Autodesk Inventor part; units mm, degrees
ref_plane "YZ Plane" through (0, 0, 0) normal (1, 0, 0) x (0, 1, 0)
ref_plane "XZ Plane" through (0, 0, 0) normal (0, 1, 0) x (-1, 0, 0)
ref_plane "XY Plane" through (0, 0, 0) normal (0, 0, 1) x (1, 0, 0)
sketch "Sketch1" plane through (0, 0, 0) normal (0, 1, 0) x (-1, 0, 0)
  line L0 (0, 0) -> (-425, 0)
  line L1 (-425, 0) -> (-425, -355)
  line L2 (-425, -355) -> (0, -355)
  line L3 (0, -355) -> (0, 0)
  line L4 (-20, -15) -> (-405, -15)
  line L5 (-405, -15) -> (-405, -340)
  line L6 (-405, -340) -> (-20, -340)
  line L7 (-20, -340) -> (-20, -15)
  dimension "d0" = 425
  dimension "d1" = 355
  dimension "d2" = 385
  dimension "d3" = 325
extrude "Extrusion1" add sketch "Sketch1" along normal blind 247
sketch "Sketch2" plane through (0, 0, 0) normal (0, -1, 0) x (1, 0, 0)
  line L0 (0, -355) -> (0, 0)
  line L1 (425, 0) -> (425, -355)
  line L2 (0, 0) -> (425, 0)
  line L3 (425, 0) -> (425, -355)
  line L4 (425, -355) -> (0, -355)
  line L5 (0, -355) -> (0, 0)
extrude "Extrusion2" add sketch "Sketch2" against normal blind 7
sketch "Sketch3" plane through (20, 247, -15) normal (1, 0, 0) x (0, 0, -1)
  line L0 (0, -240) -> (325, -240)
  line L1 (0, -240) -> (162.5, -240)
  point P0 (-15, -247)
  dimension "d8" = 162.5
sketch "Sketch4" plane through (405, 247, -340) normal (-1, 0, 0) x (0, 0, 1)
  point P0 (340, -247)
sketch "Sketch5" plane through (405, 247, -340) normal (-1, 0, 0) x (0, 0, 1)
  line L0 (325, -240) -> (0, -240)
  line L1 (325, -240) -> (162.5, -240)
  point P0 (340, -247)
sketch "Sketch6" plane through (405, 247, -340) normal (-1, 0, 0) x (0, 0, 1)
  line L0 (0, -240) -> (325, -240)
  line L1 (325, -240) -> (162.5, -240)
  point P0 (340, -247)
  dimension "d9" = 162.5
properties part number "Olkasse"
Part model, mm, in its own coordinate system. A direction names the side the tool comes from. Coordinates: 2 decimals unless noted, no trailing zeros. Order: outer loops, then holes, each group sorted by start corner. A loop starts at its lowest first (then second) coordinate and runs counter-clockwise, first axis right, second up. Notation, with made-up numbers: (29, 22) - (41, 22) arc R20 cw to (41, 56) - close; hole circle Ø8 at (0.5, -16). An arc over 180 degrees is marked (long way). Return JSON: item names as keys, results as strings. Group by question number.
Item 1: Pin check, flat tips, straight feed: pin 1 (12 mm diameter, centred on x = 320, z = -292, fed in from -Y); pin 2 (4 mm diameter, centred on x = 72, z = -171, fed in from +Y). Stop position of each tip, or through.
Item 2: Cut at A-A (y = 195). List the corners of the cut face in (x, z).
Item 3: Pull direction Z, two halves, no side cores. Call faces 1 (the face through (215, 122, -355)), 2 (the face through (229, 247, -348)), 3 (the face through (405, 125, -175)), 4 (the face through (20, 125, -180)): pulls with the +Z half, pulls with the -Z half, needs draft (parallel to the pull), parting line crosses it, or undercut.
Item 4: Cut at C-C (x = 134.5). List the corners of the cut face in (y, z).
Item 5: Drill centre lines: probe 1 along Z at (x, y) = (245, 131.5); probe 2 along X at (y, z) = (178.5, -85.5); probe 3 along Y at (x, z) = (238.5, -185). Where is each one in solid material? Low to high. Write a range as from..to.
Item 6: Which spindle directions (+Z, -Z, +X, -X, +Y, -Y) get a long thin tool onto all of the face, cutting with end or side? Do faces 5 (the face through (425, 122, -175)), 6 (the face through (215, 125, -340)). Say none if no direction does.
Item 7: Cut at B-B (z = -327). List the corners of the cut face in (x, y).
Check values:
{
 "1": {"pin 1": "stops at y = 0", "pin 2": "stops at y = 7"},
 "2": {"outline": "(0, -355) - (425, -355) - (425, 0) - (0, 0) - close; hole (20, -340) - (405, -340) - (405, -15) - (20, -15) - close"},
 "3": {"face 1": "pulls with the -Z half", "face 2": "needs draft", "face 3": "undercut", "face 4": "undercut"},
 "4": {"outline": "(0, -355) - (247, -355) - (247, -340) - (7, -340) - (7, -15) - (247, -15) - (247, 0) - (0, 0) - close"},
 "5": {"probe 1": "z = -355..-340, -15..0", "probe 2": "x = 0..20, 405..425", "probe 3": "y = 0..7"},
 "6": {"face 5": "+Z, -Z, +X, +Y, -Y", "face 6": "+Y"},
 "7": {"outline": "(0, 0) - (425, 0) - (425, 247) - (405, 247) - (405, 7) - (20, 7) - (20, 247) - (0, 247) - close"}
}
